For this review, take the finished solid that the model builds, in its own axes (mm). Face numbers are marked on the shaded views. A direction names the side the tool comes from. Round coordinates to 2 decimals unless told otherwise and drop trailing zeros. Write each loop counter-clockwise with the first axis right and the second up, starting at its lowest first coordinate (ties: lowest second). Pieces come first, ordered by that corner, then holes. Notation, with made-up numbers: M 12.25,-8 L 30.25,-8 A25 ccw 30.25,30 Z; hole C -5,82.25 d6. An arc over 180 degrees is marked long. Answer in a Markdown table with one row per item.
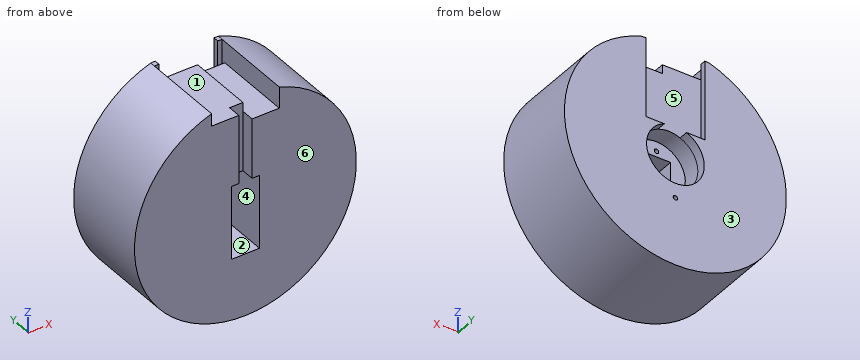
```python
from build123d import *
from build123d.topology import SkipClean

# Parameters (mm, degrees)
SKETCH7_R            = 50
SKETCH7_W            = 12.7
SKETCH7_H            = 33.05
BOSS_EXTRUDE4_DEPTH  = 19.2
SKETCH8_R            = 50
SKETCH8_W            = 12.7
SKETCH8_H            = 23.2
BOSS_EXTRUDE5_DEPTH  = 8.2
SKETCH11_R           = 50
SKETCH11_R_2         = 13
BOSS_EXTRUDE6_DEPTH  = 8.2
SKETCH12_R           = 1
CUT_EXTRUDE4_DEPTH   = 74.271003815
SKETCH13_W           = 30.5
SKETCH13_H           = 8
CUT_EXTRUDE5_DEPTH   = 35.6
CUT_EXTRUDE6_DEPTH   = 6
SKETCH15_W           = 12.25
SKETCH15_H           = 4
CUT_EXTRUDE7_DEPTH   = 29.6
SKETCH16_R           = 1
BOSS_EXTRUDE11_DEPTH = 5.2
CUT_EXTRUDE8_START   = -1
SKETCH20_R           = 50
CUT_EXTRUDE8_DEPTH   = 1
BOSS_EXTRUDE12_DEPTH = 2.4


with BuildPart() as part:
    # Sketch7 → Boss-Extrude4 (new body)
    with BuildSketch(Plane(origin=(0, 0, 0), x_dir=(1, 0, 0), z_dir=(0, 1, 0))):
        with Locations(Location((0, 0, 0), (0, 0, 270))):
            Circle(SKETCH7_R)
        with Locations((0, 5.455)):
            Rectangle(SKETCH7_W, SKETCH7_H, mode=Mode.SUBTRACT)
    extrude(amount=BOSS_EXTRUDE4_DEPTH)

    # Sketch8 → Boss-Extrude5 (add)
    with BuildSketch(Plane(origin=(0, 19.2, 0), x_dir=(1, 0, 0), z_dir=(0, 1, 0))):
        with Locations(Location((0, 0, 0), (0, 0, 270))):
            Circle(SKETCH8_R)
        with Locations((0, 5.455)):
            Rectangle(SKETCH8_W, SKETCH8_H, mode=Mode.SUBTRACT)
    extrude(amount=BOSS_EXTRUDE5_DEPTH)

    # Sketch11 → Boss-Extrude6 (add)
    with BuildSketch(Plane(origin=(0, 27.4, 0), x_dir=(1, 0, 0), z_dir=(0, 1, 0))):
        with Locations(Location((0, 0, 0), (0, 0, 270))):
            Circle(SKETCH11_R)
        with Locations(Location((0, 0, 0), (0, 0, 119.239513028))):
            Circle(SKETCH11_R_2, mode=Mode.SUBTRACT)
    extrude(amount=BOSS_EXTRUDE6_DEPTH)

    # Sketch12 → Cut-Extrude4 (cut, through all)
    with BuildSketch(Plane.XZ.offset(-19.2)):
        with Locations(Location((0, 8.67, 0), (0, 0, 270))):
            Circle(SKETCH12_R)
        with Locations(Location((0, -19.58, 0), (0, 0, 270))):
            Circle(SKETCH12_R)
    extrude(amount=-CUT_EXTRUDE4_DEPTH, mode=Mode.SUBTRACT)

    # Sketch13 → Cut-Extrude5 (cut)
    with BuildSketch(Plane.XZ):
        with Locations((0, 46)):
            Rectangle(SKETCH13_W, SKETCH13_H)
    extrude(amount=-CUT_EXTRUDE5_DEPTH, mode=Mode.SUBTRACT)

    # Sketch14 → Cut-Extrude6 (cut)
    with BuildSketch(Plane.XZ):
        Polygon((-3, 11.07), (3, 11.07), (3, 38), (15.25, 38), (15.25, 42), (3, 42), (-3, 42), align=None)
    extrude(amount=-CUT_EXTRUDE6_DEPTH, mode=Mode.SUBTRACT)

    # Sketch15 → Cut-Extrude7 (cut)
    with BuildSketch(Plane.XZ.offset(-6)):
        with Locations((9.125, 40)):
            Rectangle(SKETCH15_W, SKETCH15_H)
    extrude(amount=-CUT_EXTRUDE7_DEPTH, mode=Mode.SUBTRACT)

    # Sketch16 → Boss-Extrude11 (add)
    with BuildSketch(Plane(origin=(0, 35.6, 0), x_dir=(1, 0, 0), z_dir=(0, 1, 0))):
        with BuildLine():
            ThreePointArc((15.25, -47.617617538), (0, 50), (-15.25, -47.617617538))
            Line((-15.25, -47.617617538), (-15.25, -42))
            Line((-15.25, -42), (-15.25, -12))
            Line((-15.25, -12), (-5, -12))
            ThreePointArc((-5, -12), (-7.211102551, 10.816653826), (13, 0))
            ThreePointArc((13, 0), (10.816653826, -7.211102551), (5, -12))
            Line((5, -12), (15.25, -12))
            Line((15.25, -12), (15.25, -38))
            Line((15.25, -38), (15.25, -47.617617538))
        make_face()
        with Locations(Location((0, 19.58, 0), (0, 0, 90))):
            Circle(SKETCH16_R, mode=Mode.SUBTRACT)
    extrude(amount=BOSS_EXTRUDE11_DEPTH)

    # Sketch20 → Cut-Extrude8 (cut)
    with SkipClean():  # the faces are left unmerged after this step: merging them gives an invalid solid
        with BuildSketch(Plane(origin=(0, 40.8, 0), x_dir=(1, 0, 0), z_dir=(0, 1, 0)).offset(CUT_EXTRUDE8_START)):
            Circle(SKETCH20_R)
        extrude(amount=CUT_EXTRUDE8_DEPTH, mode=Mode.SUBTRACT)

    # Sketch21 → Boss-Extrude12 (add)
    with SkipClean():  # the faces are left unmerged after this step: merging them gives an invalid solid
        with BuildSketch(Plane(origin=(0, 39.8, 0), x_dir=(1, 0, 0), z_dir=(0, 1, 0))):
            Polygon((-15.25, -12), (-13.25, -12), (-13.25, -47.685588874), (-15.25, -47.617617538), align=None)
            Polygon((13.25, -47.685588874), (15.25, -47.617617538), (15.25, -12), (13.25, -12), align=None)
        extrude(amount=-BOSS_EXTRUDE12_DEPTH)


solid = part.part
```
Q1. Take a section at D-D (x = -30). State the section outline as (y, z) points, then the cut area to 3 significant figures.
Found:
| item | result |
|---|---|
| outline | M 0,-40 L 39.8,-40 L 39.8,40 L 0,40 Z |
| area | 3,180 mm² |
Q2. For probe 1 along Y at (x, z) = (-14, 29); probe 2 along X at (y, z) = (5, 1); probe 3 along X at (y, z) = (37, 0), list the stretches that pass through material, from the lowest coordinate up.
Found:
| item | result |
|---|---|
| probe 1 | 0 to 35.6, 37.4 to 39.8 |
| probe 2 | -49.99 to -6.35, 6.35 to 49.99 |
| probe 3 | -50 to -13, 13 to 50 |
Q3. Take a section at A-A (y = 3). State the section outline as (x, z) points, then the cut area to 3 significant figures.
Found:
| item | result |
|---|---|
| outline | M -15.25,42 L -15.25,47.62 A50 ccw long 15.25,47.62 L 15.25,38 L 3,38 L 3,11.07 L 6.35,11.07 L 6.35,-21.98 L -6.35,-21.98 L -6.35,11.07 L -3,11.07 L -3,42 Z |
| area | 6,980 mm² |
Q4. Machinability: for the marked faces 5 and 6, which of the approach directions +Z, -Z, +X, -X, +Y, -Y give a long, thin tool a straight path to every point of the face, cutting with its end or side? Answer none if there is none.
Found:
| item | result |
|---|---|
| face 5 | +Z |
| face 6 | +Z, -Z, +X, -X, -Y |
Q5. Take a section at C-C (z = 18.5). State the section outline as (x, y) points, then the cut area to 3 significant figures.
Found:
| item | result |
|---|---|
| outline | M -46.45,0 L -3,0 L -3,6 L 3,6 L 3,0 L 46.45,0 L 46.45,39.8 L 13.25,39.8 L 13.25,37.4 L 15.25,37.4 L 15.25,35.6 L -15.25,35.6 L -15.25,37.4 L -13.25,37.4 L -13.25,39.8 L -46.45,39.8 Z |
| area | 3,540 mm² |
Q6. Mouldability with a two-part tool opening along Z and no side actions: class the marked faces 1, 2, 3 and 4 as +Z half, -Z half, draft (parallel to the pull), parting line (faces both ways), or undercut.
Found:
| item | result |
|---|---|
| face 1 | +Z half |
| face 2 | undercut |
| face 3 | draft |
| face 4 | undercut |
Q7. Take a section at B-B (x = -8). State the section outline as (y, z) points, then the cut area to 3 significant figures.
Found:
| item | result |
|---|---|
| outline | M 0,-49.36 L 39.8,-49.36 L 39.8,-10.25 L 27.4,-10.25 L 27.4,10.25 L 39.8,10.25 L 39.8,12 L 35.6,12 L 35.6,42 L 0,42 Z |
| area | 3,260 mm² |
Q8. Insertion check: P1, Ø3, axis at x = -4.5, y = 25, coming from the -Z side; P2, Ø8, axis at y = 13, z = -6.5, coming from the -X side; P3, Ø4, axis at x = -23, z = -18.5, coming from the -Y side; P4, Ø3, axis at x = -2.5, z = -14.5, coming from the -Y side. Each pin has a flat end and moves straight along its axis. Give the tip position at first contact, or say it passes through.
Found:
| item | result |
|---|---|
| P1 | z = -49.91 |
| P2 | x = -49.94 |
| P3 | y = 0 |
| P4 | y = 27.4 |
